Job drawing, mm, ordinate dimensions from the low corner. One solid piece. Coordinates: 2 decimals unless noted, no trailing zeros. Loops run counter-clockwise (first coordinate to the right, second up) from the corner with the lowest first, then second, coordinate; pieces in that order, holes last. Notation, with made-up numbers: (5.25, -2.75) -> (44.25, -2.75) arc R21 ccw to (44.25, 10.25) -> close; hole circle Ø1 at (17.5, -16). An arc over 180 degrees is marked (long way). Use one line per item in the form item = value. Start each with the question number.
(1) Drill centre lines: L1, parallel to Y at x = 10, z = 7; L2, parallel to X at y = 90.5, z = 5; L3, parallel to X at y = 81, z = 5. Where is each one in solid material? Low to high. Write a range as [from, to].
(2) Pin check, flat tips, straight feed: P1, Ø3.5, axis at x = 22, z = 5, coming from the -Y side; P2, Ø1.2, axis at x = 22.5, z = 4.5, coming from the +Y side. Stop position of each tip, or through.
(3) Band-saw the part on C-C on z = 5. Give the cut face in (x, y).
(4) Band-saw the part on B-B on x = 10. Give the cut face in (y, z), then the cut area to 3 significant figures.
(5) Band-saw the part on A-A on y = 79. Give the cut face in (x, z).
(6) Mould opens along Y. For the marked faces 1, 2, 3 and 4 say: +Y half, -Y half, draft (parallel to the pull), parting line (faces both ways), or undercut.
(7) Band-saw the part on D-D on y = 49. Give the cut face in (x, z).
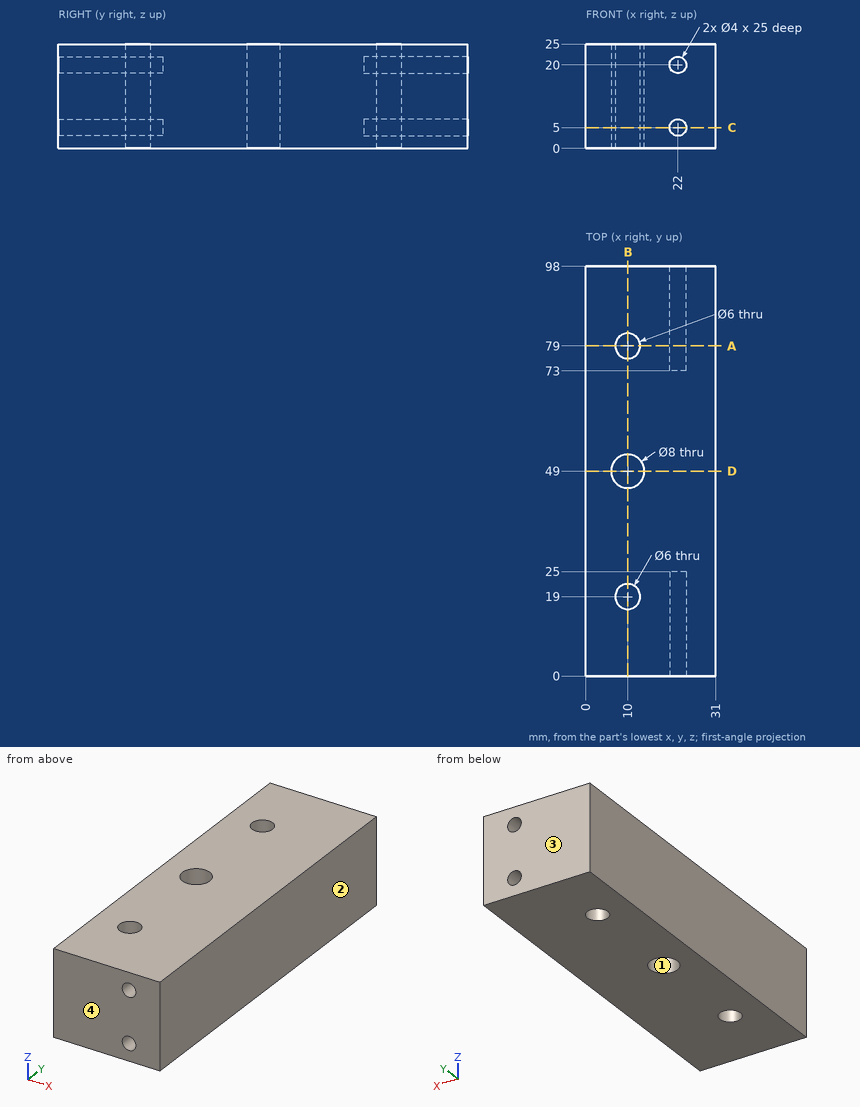
A:
q1.L1 = [0, 16], [22, 45], [53, 76], [82, 98]
q1.L2 = [0, 20], [24, 31]
q1.L3 = [0, 7.76], [12.24, 20], [24, 31]
q2.P1 = 25
q2.P2 = 73
q3.outline = (0, 0) -> (20, 0) -> (20, 25) -> (24, 25) -> (24, 0) -> (31, 0) -> (31, 98) -> (24, 98) -> (24, 73) -> (20, 73) -> (20, 98) -> (0, 98) -> close; hole circle Ø8 at (10, 49); hole circle Ø6 at (10, 19); hole circle Ø6 at (10, 79)
q4.outline = (0, 0) -> (16, 0) -> (16, 25) -> (0, 25) -> close; (22, 0) -> (45, 0) -> (45, 25) -> (22, 25) -> close; (53, 0) -> (76, 0) -> (76, 25) -> (53, 25) -> close; (82, 0) -> (98, 0) -> (98, 25) -> (82, 25) -> close
q4.area = 1,950 mm²
q5.outline = (0, 0) -> (7, 0) -> (7, 25) -> (0, 25) -> close; (13, 0) -> (31, 0) -> (31, 25) -> (13, 25) -> close; hole circle Ø4 at (22, 5); hole circle Ø4 at (22, 20)
q6.face_1 = undercut
q6.face_2 = draft
q6.face_3 = +Y half
q6.face_4 = -Y half
q7.outline = (0, 0) -> (6, 0) -> (6, 25) -> (0, 25) -> close; (14, 0) -> (31, 0) -> (31, 25) -> (14, 25) -> close
